For this review, use the dimensioned drawing (mm, ordinates from the lowest corner) and the shaded views. Round coordinates to 2 decimals unless told otherwise and drop trailing zeros. Loops run counter-clockwise (first coordinate to the right, second up) from the corner with the lowest first, then second, coordinate; pieces in that order, holes last. Notation, with made-up numbers: (-9, 88.5) - (23, 88.5) arc R23 ccw to (23, 106.5) - close; hole circle Ø1 at (46, -2.5). An arc over 180 degrees is marked (long way). Use one line per item in the form item = value. Start each with the question number.
(1) We need section B-B, the plane z = 15.5. Write out the cut boundary in (x, y) (1 decimal).
(2) We need section A-A, the plane x = 25.4. Write out the cut boundary in (y, z).
(3) We need section D-D, the plane y = 0.6. Write out the cut boundary in (x, z).
(4) We need section C-C, the plane x = 20. Write out the cut boundary in (y, z).
(5) Wall thickness on probe 1 along Z at (x, y) = (25.4, 1.75); probe 2 along Z at (x, y) = (35.3, 1.7) (1 decimal); probe 3 along X at (y, z) = (1.1, 17) (1 decimal): over which ranges is each line inside the solid? List them lowest first. Write a range as [from, to].
(6) For pin 1 (5 mm diameter, centred on x = 25.4, z = 4.75, fed in from -Y); pin 2 (3.5 mm diameter, centred on x = 15.5, z = 35.3, fed in from -Y); pin 3 (1 mm diameter, centred on y = 1.5, z = 34, fed in from +X), all flat-tipped, find the tip position at first contact; note any pin that passes through.
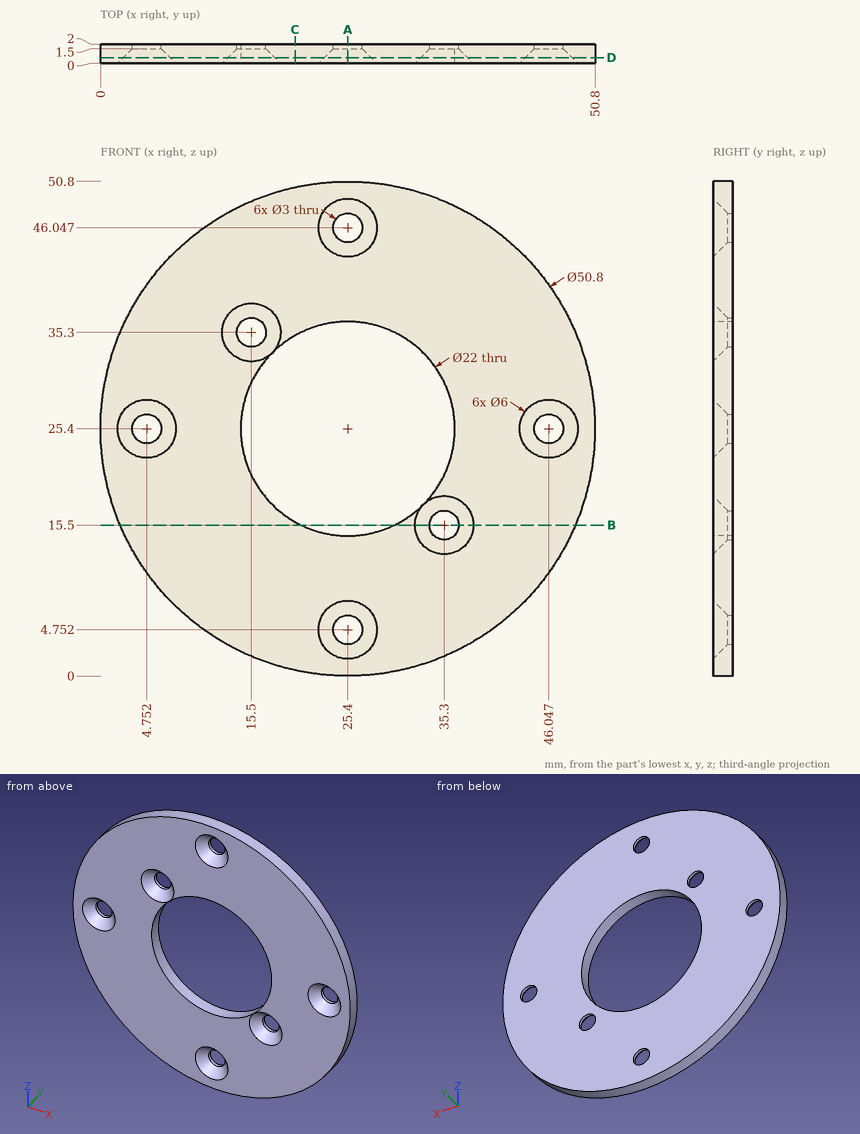
Data:
q1.outline = (2, 0) - (20.6, 0) - (20.6, 2) - (2, 2) - close; (30.2, 0) - (32.3, 0) - (33.8, 1.5) - (33.8, 2) - (30.2, 2) - close; (36.8, 1.5) - (38.3, 0) - (48.8, 0) - (48.8, 2) - (36.8, 2) - close
q2.outline = (0, 0) - (2, 0) - (2, 3.25) - (1.5, 3.25) - (0, 1.75) - close; (0, 7.75) - (1.5, 6.25) - (2, 6.25) - (2, 14.4) - (0, 14.4) - close; (0, 36.4) - (2, 36.4) - (2, 44.55) - (1.5, 44.55) - (0, 43.05) - close; (0, 49.05) - (1.5, 47.55) - (2, 47.55) - (2, 50.8) - (0, 50.8) - close
q3.outline = circle Ø50.8 at (25.4, 25.4); hole circle Ø4.8 at (4.75, 25.4); hole circle Ø4.8 at (15.5, 35.3); hole circle Ø22 at (25.4, 25.4); hole circle Ø4.8 at (25.4, 4.75); hole circle Ø4.8 at (25.4, 46.05); hole circle Ø4.8 at (35.3, 15.5); hole circle Ø4.8 at (46.05, 25.4)
q4.outline = (0, 0.58) - (2, 0.58) - (2, 15.82) - (0, 15.82) - close; (0, 34.98) - (2, 34.98) - (2, 50.22) - (0, 50.22) - close
q5.probe_1 = [0, 3.25], [6.25, 14.4], [36.4, 44.55], [47.55, 50.8]
q5.probe_2 = [2, 14], [17, 20.6], [30.2, 48.8]
q5.probe_3 = [1.4, 18.3], [32.5, 34.1], [36.5, 49.4]
q6.pin_1 = 0.5
q6.pin_2 = 1.25
q6.pin_3 = 49.47
